Input: part model. Units: mm. Frame: model coordinates. A direction names the side the tool comes from. Coordinates: 2 decimals unless noted, no trailing zeros. Write each loop counter-clockwise with the first axis right and the second up, starting at its lowest first coordinate (ties: lowest second). Pieces come first, ordered by that corner, then holes. Notation, with made-up numbers: (14.25, -21.75) - (45.25, -21.75) arc R26 ccw to (45.25, 12.25) - close; hole circle Ø8 at (56.5, -7.75). An arc over 180 degrees is marked (long way). One line per question, with ' | ' between items. Start each with the question number.
1) First-contact query: P1, Ø1, axis at x = -2, z = -3.5, coming from the -Y side. Flat tip, straight axial feed; report the tip coordinate or a pass-through.
2) Draft query along Y for faces 6 (the flat face through (-15, 55, -2)), 7 (the cylindrical face through (24, 73, 2)), 8 (the cylindrical face through (-5.1, 67.4, 1.5)), 9 (the cylindrical face through (23, 1, 2)). Return one class per face: released by +Y, released by -Y, zero draft, split by the parting line, or undercut.
3) Section query D-D on x = -5.5. Return loops of the section in (y, z) (3 decimals).
4) Reachability of faces 1 (the flat face through (17.625, 25.304, 6.141)), 2 (the flat face through (25, 37, 0)), 3 (the cylindrical face through (11.61, 38.89, -1.81)), 4 (the cylindrical face through (14.681, 42.722, 6.234)), 5 (the flat face through (19, 42.5, 6)) from +Z, -Z, +X, -X, +Y, -Y: full face, straight path, thin tool, end or side. Return the list, or none.
5) Section query A-A on z = 7.5. Return loops of the section in (x, y), and give its area (3 significant figures).
6) Section query C-C on y = 37.5. Return loops of the section in (x, z), and give its area (3 significant figures).
7) Section query B-B on z = 0.75. Return loops of the section in (x, y), and give its area (3 significant figures).
8) Line query: line 1 (Y direction, x = 12.5, z = -2); line 2 (X direction, y = 69, z = -1.75); line 3 (X direction, y = 69, z = 3.5). Output: solid intervals per line, ascending.
```python
from build123d import *
from build123d.topology import SkipClean

# Parameters (mm, degrees)
SKETCH1_R           = 1.5
SKETCH1_W           = 15
SKETCH1_H           = 37.5
BOSS_EXTRUDE1_DEPTH = 2.85
FILLET1_R           = 5
FILLET2_R           = 2
BOSS_EXTRUDE2_START = 3.5
SKETCH5_R           = 1.5
BOSS_EXTRUDE2_DEPTH = 3.5
FILLET3_R           = 3.5
FILLET4_R           = 2
FILLET5_R           = 2
SKETCH6_R           = 1.5
CUT_EXTRUDE1_DEPTH  = 10
SKETCH8_R           = 1.5
BOSS_EXTRUDE3_DEPTH = 6.35
BOSS_EXTRUDE4_START = 3.175
SKETCH9_R           = 1.5
BOSS_EXTRUDE4_DEPTH = 3.175
SKETCH10_W          = 40
SKETCH10_H          = 15.399494937
SKETCH10_W_2        = 25
BOSS_EXTRUDE5_DEPTH = 6.675
CUT_EXTRUDE2_START  = -6.675
CUT_EXTRUDE2_DEPTH  = 6.675
BOSS_EXTRUDE6_START = -9.2
BOSS_EXTRUDE6_DEPTH = 9.2
FILLET6_R           = 7
BOSS_EXTRUDE7_DEPTH = 6.675
FILLET7_R           = 3
FILLET8_R           = 1.5
SKETCH15_R          = 1.65
CUT_EXTRUDE3_DEPTH  = 81.63507689


# Read off the part's stored shape, not the designer's step: Cut-Extrude2
with BuildPart() as part:
    # Sketch1 → Boss-Extrude1 (new body)
    # profile 1 of 2: a face of its own
    with BuildSketch(Plane.XY):
        Polygon((0, 37.5), (0, 0), (25, 0), (25, 75), (0, 75), align=None)
        with Locations((12.5, 6)):
            Circle(SKETCH1_R, mode=Mode.SUBTRACT)
        with Locations((12.5, 37.5)):
            Circle(SKETCH1_R, mode=Mode.SUBTRACT)
        with Locations((12.5, 69)):
            Circle(SKETCH1_R, mode=Mode.SUBTRACT)
    # profile 2 of 2: a face of its own
    with BuildSketch(Plane.XY):
        with Locations((-7.5, 56.25)):
            Rectangle(SKETCH1_W, SKETCH1_H)
    extrude(amount=BOSS_EXTRUDE1_DEPTH)

    # Fillet1
    fillet1_edges = [part.edges().sort_by_distance(p)[0] for p in [
        (25, 75, 1.425),
        (25, 0, 1.425),
        (0, 0, 1.425),
        (0, 37.5, 1.425),
        (-15, 75, 1.425),
    ]]
    fillet(fillet1_edges, radius=FILLET1_R)

    # Fillet2
    fillet2_edges = [part.edges().sort_by_distance(p)[0] for p in [
        (-15, 37.5, 1.425),
    ]]
    fillet(fillet2_edges, radius=FILLET2_R)

    # Sketch5 → Boss-Extrude2 (add)
    # profile 1 of 2: a face of its own
    with BuildSketch(Plane.XY.offset(2.85).offset(BOSS_EXTRUDE2_START)):
        with BuildLine():
            Line((-15, 42.5), (10.428932188, 42.5))
            Line((10.428932188, 42.5), (21.464466094, 53.535533906))
            Line((21.464466094, 53.535533906), (25, 57.071067812))
            Line((25, 57.071067812), (25, 70))
            ThreePointArc((25, 70), (23.535533906, 73.535533906), (20, 75))
            Line((20, 75), (-10, 75))
            ThreePointArc((-10, 75), (-13.535533906, 73.535533906), (-15, 70))
            Line((-15, 70), (-15, 42.5))
        make_face()
        with Locations((12.5, 69)):
            Circle(SKETCH5_R, mode=Mode.SUBTRACT)
    # profile 2 of 2: a face of its own
    with BuildSketch(Plane.XY.offset(2.85).offset(BOSS_EXTRUDE2_START)):
        with BuildLine():
            Line((14.571067812, 32.5), (0, 17.928932188))
            Line((0, 17.928932188), (0, 5))
            ThreePointArc((0, 5), (1.464466094, 1.464466094), (5, 0))
            Line((5, 0), (20, 0))
            ThreePointArc((20, 0), (23.535533906, 1.464466094), (25, 5))
            Line((25, 5), (25, 32.5))
            Line((25, 32.5), (14.571067812, 32.5))
        make_face()
        with Locations((12.5, 6)):
            Circle(SKETCH5_R, mode=Mode.SUBTRACT)
    extrude(amount=-BOSS_EXTRUDE2_DEPTH)

    # Fillet3
    fillet3_edges = [part.edges().sort_by_distance(p)[0] for p in [
        (10.428932188, 42.5, 4.6),
        (14.571067812, 32.5, 4.6),
    ]]
    fillet(fillet3_edges, radius=FILLET3_R)

    # Fillet4
    fillet4_edges = [part.edges().sort_by_distance(p)[0] for p in [
        (-15, 42.5, 4.6),
    ]]
    fillet(fillet4_edges, radius=FILLET4_R)

    # Fillet5
    fillet5_edges = [part.edges().sort_by_distance(p)[0] for p in [
        (25, 57.071067812, 4.6),
        (25, 32.5, 4.6),
        (0, 17.928932188, 4.6),
    ]]
    fillet(fillet5_edges, radius=FILLET5_R)

    # Sketch6 → Cut-Extrude1 (cut)
    with BuildSketch(Plane.XY.offset(6.35)):
        with Locations((-5.5, 69)):
            Circle(SKETCH6_R)
    extrude(amount=-CUT_EXTRUDE1_DEPTH, mode=Mode.SUBTRACT)

    # Sketch8 → Boss-Extrude3 (add)
    with SkipClean():  # the faces are left unmerged after this step: merging them gives an invalid solid
        with BuildSketch(Plane(origin=(0, 0, 0), x_dir=(-1, 0, 0), z_dir=(0, 0, -1))):
            with BuildLine():
                ThreePointArc((0, 32.5), (1.464466094, 36.035533906), (5, 37.5))
                Line((5, 37.5), (13, 37.5))
                ThreePointArc((13, 37.5), (14.414213562, 38.085786438), (15, 39.5))
                Line((15, 39.5), (15, 70))
                ThreePointArc((15, 70), (13.535533906, 73.535533906), (10, 75))
                Line((10, 75), (-20, 75))
                ThreePointArc((-20, 75), (-23.535533906, 73.535533906), (-25, 70))
                Line((-25, 70), (-25, 5))
                ThreePointArc((-25, 5), (-23.535533906, 1.464466094), (-20, 0))
                Line((-20, 0), (-5, 0))
                ThreePointArc((-5, 0), (-1.464466094, 1.464466094), (0, 5))
                Line((0, 5), (0, 32.5))
            make_face()
            with Locations((-12.5, 6)):
                Circle(SKETCH8_R, mode=Mode.SUBTRACT)
            with Locations((-12.5, 69)):
                Circle(SKETCH8_R, mode=Mode.SUBTRACT)
            with Locations((-12.5, 37.5)):
                Circle(SKETCH8_R, mode=Mode.SUBTRACT)
            with Locations(Location((5.5, 69, 0), (0, 0, 180))):
                Circle(SKETCH8_R, mode=Mode.SUBTRACT)
        extrude(amount=BOSS_EXTRUDE3_DEPTH)
    add(part.part.scale(1), mode=Mode.REPLACE)  # the faces are merged on a copy

    # Sketch9 → Boss-Extrude4 (add)
    # profile 1 of 2: a face of its own
    with BuildSketch(Plane.XY.offset(6.35).offset(BOSS_EXTRUDE4_START)):
        with BuildLine():
            ThreePointArc((16.02081528, 32.5), (14.681423267, 32.233578364), (13.545941546, 31.474873734))
            Line((13.545941546, 31.474873734), (0.585786438, 18.514718626))
            ThreePointArc((0.585786438, 18.514718626), (0.152240935, 17.865871928), (0, 17.100505063))
            Line((0, 17.100505063), (0, 5))
            ThreePointArc((0, 5), (1.464466094, 1.464466094), (5, 0))
            Line((5, 0), (20, 0))
            ThreePointArc((20, 0), (23.535533906, 1.464466094), (25, 5))
            Line((25, 5), (25, 30.5))
            ThreePointArc((25, 30.5), (24.414213562, 31.914213562), (23, 32.5))
            Line((23, 32.5), (16.02081528, 32.5))
        make_face()
    # profile 2 of 2: a face of its own
    with BuildSketch(Plane.XY.offset(6.35).offset(BOSS_EXTRUDE4_START)):
        with BuildLine():
            ThreePointArc((8.97918472, 42.5), (10.318576733, 42.766421636), (11.454058454, 43.525126266))
            Line((11.454058454, 43.525126266), (24.414213562, 56.485281374))
            ThreePointArc((24.414213562, 56.485281374), (24.847759065, 57.134128072), (25, 57.899494937))
            Line((25, 57.899494937), (25, 70))
            ThreePointArc((25, 70), (23.535533906, 73.535533906), (20, 75))
            Line((20, 75), (-10, 75))
            ThreePointArc((-10, 75), (-13.535533906, 73.535533906), (-15, 70))
            Line((-15, 70), (-15, 44.5))
            ThreePointArc((-15, 44.5), (-14.414213562, 43.085786438), (-13, 42.5))
            Line((-13, 42.5), (8.97918472, 42.5))
        make_face()
        with Locations((-5.5, 69)):
            Circle(SKETCH9_R, mode=Mode.SUBTRACT)
        with Locations((12.5, 69)):
            Circle(SKETCH9_R, mode=Mode.SUBTRACT)
    extrude(amount=-BOSS_EXTRUDE4_DEPTH)

    # Sketch10 → Boss-Extrude5 (add)
    with SkipClean():  # the faces are left unmerged after this step: merging them gives an invalid solid
        with BuildSketch(Plane.XY.offset(9.525)):
            with Locations((5, 50.199747469)):
                Rectangle(SKETCH10_W, SKETCH10_H)
            with Locations((12.5, 24.800252531)):
                Rectangle(SKETCH10_W_2, SKETCH10_H)
        extrude(amount=-BOSS_EXTRUDE5_DEPTH)

    # Cut-Extrude2 outline → Cut-Extrude2 (cut)
    with SkipClean():  # the faces are left unmerged after this step: merging them gives an invalid solid
        with BuildSketch(Plane.XY.offset(9.525).offset(CUT_EXTRUDE2_START)):
            Polygon((25, 32.5), (10.428932188, 32.5), (25, 17.928932188), align=None)
            with BuildLine():
                Line((-15, 42.5), (14.571067812, 42.5))
                Line((14.571067812, 42.5), (-14.682437359, 71.75350517))
                ThreePointArc((-14.682437359, 71.75350517), (-14.919968841, 70.891014367), (-15, 70))
                Line((-15, 70), (-15, 42.5))
            make_face()
        extrude(amount=CUT_EXTRUDE2_DEPTH, mode=Mode.SUBTRACT)

    # Sketch12 → Boss-Extrude6 (add)
    with BuildSketch(Plane(origin=(0, 0, -6.35), x_dir=(-1, 0, 0), z_dir=(0, 0, -1)).offset(BOSS_EXTRUDE6_START)):
        with BuildLine():
            Line((0, 0), (14.867488321, 38.784117768))
            ThreePointArc((14.867488321, 38.784117768), (14.133189202, 37.852006604), (13, 37.5))
            Line((13, 37.5), (5, 37.5))
            ThreePointArc((5, 37.5), (1.464466094, 36.035533906), (0, 32.5))
            Line((0, 32.5), (0, 5))
            ThreePointArc((0, 5), (-1.464466094, 1.464466094), (-5, 0))
            Line((-5, 0), (0, 0))
        make_face()
    extrude(amount=BOSS_EXTRUDE6_DEPTH)

    # Fillet6
    fillet6_edges = [part.edges().sort_by_distance(p)[0] for p in [
        (0, 0, -1.75),
    ]]
    fillet(fillet6_edges, radius=FILLET6_R)

    # Sketch13 → Boss-Extrude7 (add)
    with SkipClean():  # the faces are left unmerged after this step: merging them gives an invalid solid
        with BuildSketch(Plane.XY.offset(9.525)):
            with BuildLine():
                Line((0, 32.5), (0, 5))
                ThreePointArc((0, 5), (1.464466094, 1.464466094), (5, 0))
                Line((5, 0), (4.813322939, 0))
                ThreePointArc((4.813322939, 0), (0.847160732, 1.232023115), (-1.722886185, 4.494412187))
                Line((-1.722886185, 4.494412187), (-12.458537109, 32.5))
                Line((-12.458537109, 32.5), (0, 32.5))
            make_face()
        extrude(amount=-BOSS_EXTRUDE7_DEPTH)

    # Fillet7
    fillet7_edges = [part.edges().sort_by_distance(p)[0] for p in [
        (25, 42.5, 6.1875),
        (14.571067812, 42.5, 6.1875),
        (-14.682437359, 71.75350517, 4.6),
        (10.428932188, 32.5, 6.1875),
        (25, 17.928932188, 6.1875),
    ]]
    fillet(fillet7_edges, radius=FILLET7_R)

    # Fillet8
    # the kernel refuses this fillet: 1.5 mm, written as the material it takes off along each edge
    with BuildSketch(Plane(origin=(-12.458537109, 32.5, 14.978612885), x_dir=(0.35794111613384066, -0.9337441605605148, 0), z_dir=(0, 0, -1))) as fillet8_piece_1:
        with BuildLine():
            CenterArc((FILLET8_R * 1.45429676938, -FILLET8_R), FILLET8_R, 90, 110.97380664)
            Line((FILLET8_R * 0.520552608823, -FILLET8_R * 1.35794111613), (0, 0))
            Line((0, 0), (FILLET8_R * 1.45429676938, 0))
        make_face()
    extrude(amount=12.128612885, mode=Mode.SUBTRACT)

    # Sketch15 → Cut-Extrude3 (cut, through all)
    with BuildSketch(Plane(origin=(0, 0, -6.35), x_dir=(-1, 0, 0), z_dir=(0, 0, -1))):
        with Locations((-12.5, 69)):
            Circle(SKETCH15_R)
        with Locations((-12.5, 37.5)):
            Circle(SKETCH15_R)
        with Locations((-12.5, 6)):
            Circle(SKETCH15_R)
        with Locations((5.5, 69)):
            Circle(SKETCH15_R)
    extrude(amount=-CUT_EXTRUDE3_DEPTH, mode=Mode.SUBTRACT)


solid = part.part
```
Answer key:
1) P1: y = 3.98
2) face 6: zero draft | face 7: released by +Y | face 8: undercut | face 9: released by -Y
3) outline: (14.348, -6.35) - (67.35, -6.35) - (67.35, 9.525) - (62.571, 9.525) - (62.571, 2.85) - (32.5, 2.85) - (32.5, 9.525) - (14.348, 9.525) - close; (70.65, -6.35) - (75, -6.35) - (75, 9.525) - (70.65, 9.525) - close
4) face 1: +Z, +X | face 2: +Z, -Z, +X, +Y, -Y | face 3: +Z, -Z | face 4: +Z, -X | face 5: +Z, +X, -X
5) outline: (-12.72, 69.79) - (13.69, 43.38) arc R3 ccw to (15.81, 42.5) - (22, 42.5) arc R3 ccw to (25, 45.5) - (25, 70) arc R5 ccw to (20, 75) - (-10, 75) arc R5 ccw to (-11.49, 74.77) arc R3 ccw to start; (-11.68, 30.46) - (-1.72, 4.49) arc R7 ccw to (4.81, 0) - (20, 0) arc R5 ccw to (25, 5) - (25, 16.69) arc R3 ccw to (24.12, 18.81) - (11.31, 31.62) arc R3 ccw to (9.19, 32.5) - (-10.28, 32.5) arc R1.5 ccw to start; hole circle Ø3.3 at (-5.5, 69); hole circle Ø3.3 at (12.5, 6); hole circle Ø3.3 at (12.5, 69) | area: 1,720 mm²
6) outline: (-14.38, -6.35) - (10.85, -6.35) - (10.85, 2.85) - (-14.38, 2.85) - close; (14.15, -6.35) - (25, -6.35) - (25, 2.85) - (14.15, 2.85) - close | area: 332 mm²
7) outline: (-15, 39.5) arc R2 ccw to (-14.87, 38.78) - (-1.72, 4.49) arc R7 ccw to (4.81, 0) - (20, 0) arc R5 ccw to (25, 5) - (25, 70) arc R5 ccw to (20, 75) - (-10, 75) arc R5 ccw to (-15, 70) - close; hole circle Ø3.3 at (-5.5, 69); hole circle Ø3.3 at (12.5, 6); hole circle Ø3.3 at (12.5, 37.5); hole circle Ø3.3 at (12.5, 69) | area: 2,650 mm²
8) line 1: 0 to 4.35, 7.65 to 35.85, 39.15 to 67.35, 70.65 to 75 | line 2: -15 to -7.15, -3.85 to 10.85, 14.15 to 25 | line 3: -11.93 to -7.15, -3.85 to 10.85, 14.15 to 25
